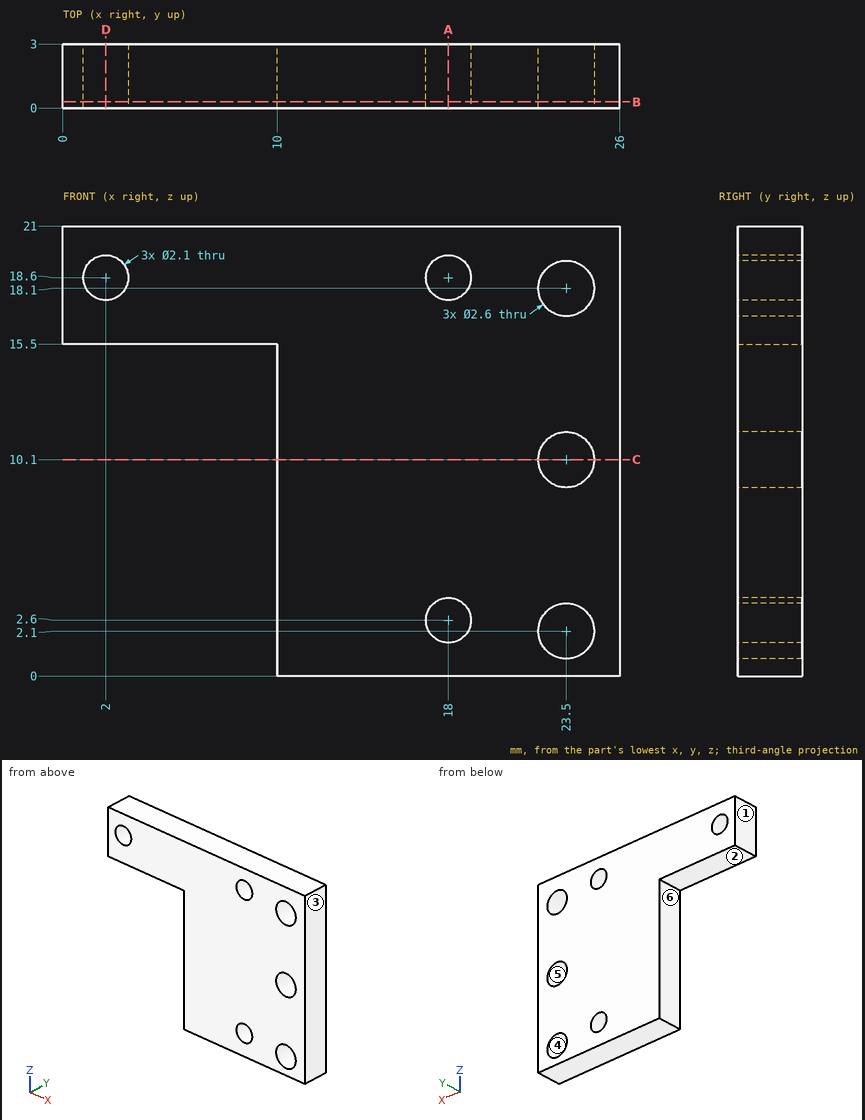
The drawing under review shows one solid part. Ordinate dimensions are in mm from its lowest x, y, z. A direction names the side the tool comes from. Coordinates: 2 decimals unless noted, no trailing zeros. Order: outer loops, then holes, each group sorted by start corner. A loop starts at its lowest first (then second) coordinate and runs counter-clockwise, first axis right, second up. Notation, with made-up numbers: (26.25, 51.25) -> (79.25, 51.25) arc R24 ccw to (79.25, 88.25) -> close; hole circle Ø5 at (66, 66.25). An arc over 180 degrees is marked (long way). Answer in a Markdown table with one row per item. Add a question column.
Item 1: We need section A-A on x = 18. Write out the cut boundary in (y, z).
Item 2: We need section D-D on x = 2. Write out the cut boundary in (y, z).
Item 3: We need section C-C on z = 10.1. Write out the cut boundary in (x, y).
Item 4: To check wall thickness, follow probe 1 along Z at (x, y) = (18, 0.8); probe 2 along X at (y, z) = (2.75, 6.75); probe 3 along X at (y, z) = (0.6, 9.25). State the ranges of each line that lie inside material, in increasing order.
Item 5: Mouldability with a two-part tool opening along X and no side actions: class the marked faces 3, 4, 5 and 6 as +X half, -X half, draft (parallel to the pull), parting line (faces both ways), or undercut.
Item 6: Clearance check with flat-ended pins moving along their axes: pin 1 (1.5 mm diameter, centred on y = 2.5, z = 15, fed in from -X); pin 2 (0.9 mm diameter, centred on y = 2, z = 8.5, fed in from -X); pin 3 (0.9 mm diameter, centred on x = 5.5, y = 1.5, fed in from -Z). State where each tip first meets the part, or that it passes through.
Item 7: We need section B-B on y = 0.3. Write out the cut boundary in (x, z), plus the area to 3 significant figures.
Item 8: Machinability: for the marked faces 1 and 2, which of the approach directions +Z, -Z, +X, -X, +Y, -Y give a long, thin tool a straight path to every point of the face, cutting with its end or side? Answer none if there is none.
Final values:
| question | item | result |
|---|---|---|
| 1 | outline | (0, 0) -> (3, 0) -> (3, 1.55) -> (0, 1.55) -> close; (0, 3.65) -> (3, 3.65) -> (3, 17.55) -> (0, 17.55) -> close; (0, 19.65) -> (3, 19.65) -> (3, 21) -> (0, 21) -> close |
| 2 | outline | (0, 15.5) -> (3, 15.5) -> (3, 17.55) -> (0, 17.55) -> close; (0, 19.65) -> (3, 19.65) -> (3, 21) -> (0, 21) -> close |
| 3 | outline | (10, 0) -> (22.2, 0) -> (22.2, 3) -> (10, 3) -> close; (24.8, 0) -> (26, 0) -> (26, 3) -> (24.8, 3) -> close |
| 4 | probe 1 | z = 0 to 1.55, 3.65 to 17.55, 19.65 to 21 |
| 4 | probe 2 | x = 10 to 26 |
| 4 | probe 3 | x = 10 to 22.52, 24.48 to 26 |
| 5 | face 3 | +X half |
| 5 | face 4 | undercut |
| 5 | face 5 | undercut |
| 5 | face 6 | -X half |
| 6 | pin 1 | stops at x = 0 |
| 6 | pin 2 | stops at x = 10 |
| 6 | pin 3 | stops at z = 15.5 |
| 7 | outline | (0, 15.5) -> (10, 15.5) -> (10, 0) -> (26, 0) -> (26, 21) -> (0, 21) -> close; hole circle Ø2.1 at (2, 18.6); hole circle Ø2.1 at (18, 2.6); hole circle Ø2.1 at (18, 18.6); hole circle Ø2.6 at (23.5, 2.1); hole circle Ø2.6 at (23.5, 10.1); hole circle Ø2.6 at (23.5, 18.1) |
| 7 | area | 365 mm2 |
| 8 | face 1 | +Z, -Z, -X, +Y, -Y |
| 8 | face 2 | -Z, -X, +Y, -Y |
